from build123d import *

# Parameters (mm, degrees)
ESQUISSE1_R        = 1.6
BOSS_EXTRU_1_DEPTH = 5


with BuildPart() as part:
    # Esquisse1 → Boss.-Extru.1 (new body)
    with BuildSketch(Plane(origin=(0, 0, 0), x_dir=(-1, 0, 0), z_dir=(0, 0, -1))):
        with BuildLine():
            Line((-34.923591431, 50.185646262), (-34.593521354, 46.781705469))
            Line((-34.593521354, 46.781705469), (-33.97698121, 43.895774796))
            Line((-33.97698121, 43.895774796), (-33.105501007, 41.345514202))
            Line((-33.105501007, 41.345514202), (-31.977290744, 38.953213644))
            Line((-31.977290744, 38.953213644), (-31.383990606, 37.884363395))
            Line((-31.383990606, 37.884363395), (-30.617930427, 37.00766319))
            Line((-30.617930427, 37.00766319), (-29.575780184, 36.488623069))
            Line((-29.575780184, 36.488623069), (-28.414519914, 36.40541305))
            Line((-28.414519914, 36.40541305), (-27.309019656, 36.770573135))
            ThreePointArc((-27.309019656, 36.770573135), (-17.618450893, 31.41303394), (-26.770699625, 25.180322464))
            Line((-26.770699625, 25.180322464), (-28.005176529, 25.48125594))
            Line((-28.005176529, 25.48125594), (-29.206336809, 25.243975885))
            Line((-29.206336809, 25.243975885), (-30.212657043, 24.546555722))
            Line((-30.212657043, 24.546555722), (-30.856527193, 23.50514548))
            Line((-30.856527193, 23.50514548), (-32.12730749, 19.451734535))
            Line((-32.12730749, 19.451734535), (-33.010967696, 15.362733581))
            Line((-33.010967696, 15.362733581), (-33.301107763, 13.363943115))
            Line((-33.301107763, 13.363943115), (-33.187947737, 12.109172823))
            Line((-33.187947737, 12.109172823), (-32.569567593, 11.011512567))
            Line((-32.569567593, 11.011512567), (-31.555037356, 10.264542393))
            Line((-31.555037356, 10.264542393), (-30.323257069, 10.000002331))
            Line((-30.323257069, 10.000002331), (-21.600005036, 10.000002331))
            ThreePointArc((-21.600005036, 10.000002331), (-21.246451562, 10.146448975), (-21.100004919, 10.500002448))
            Line((-21.100004919, 10.500002448), (-21.100004919, 14.000002331))
            Line((-21.100004919, 14.000002331), (-22.250004919, 14.000002331))
            ThreePointArc((-22.250004919, 14.000002331), (-22.676781614, 13.823225636), (-22.500004919, 14.250002331))
            Line((-22.500004919, 14.250002331), (-22.500004919, 16.250002331))
            ThreePointArc((-22.500004919, 16.250002331), (-22.676781614, 16.676779027), (-22.250004919, 16.500002331))
            Line((-22.250004919, 16.500002331), (-21.100004919, 16.500002331))
            Line((-21.100004919, 16.500002331), (-21.100004919, 17.750004196))
            ThreePointArc((-21.100004919, 17.750004196), (-21.276780955, 18.176781551), (-20.850004919, 18.000002331))
            Line((-20.850004919, 18.000002331), (-18.450004919, 18.000002331))
            ThreePointArc((-18.450004919, 18.000002331), (-18.023228224, 18.176779027), (-18.200004919, 17.750002331))
            Line((-18.200004919, 17.750002331), (-18.200004919, 16.500002331))
            Line((-18.200004919, 16.500002331), (-17.15000394, 16.500002331))
            ThreePointArc((-17.15000394, 16.500002331), (-16.763072854, 16.709167045), (-16.800004919, 16.270873119))
            Line((-16.800004919, 16.270873119), (-16.800004919, 14.250002331))
            ThreePointArc((-16.800004919, 14.250002331), (-16.623228224, 13.823225636), (-17.050004919, 14.000002331))
            Line((-17.050004919, 14.000002331), (-18.200004919, 14.000002331))
            Line((-18.200004919, 14.000002331), (-18.200004919, 10.500002448))
            ThreePointArc((-18.200004919, 10.500002448), (-18.053558275, 10.146448975), (-17.700004802, 10.000002331))
            Line((-17.700004802, 10.000002331), (-13.900003182, 10.000002331))
            ThreePointArc((-13.900003182, 10.000002331), (-13.473226487, 10.176779027), (-13.650003182, 9.750002331))
            Line((-13.650003182, 9.750002331), (-13.650003182, 0.500000117))
            ThreePointArc((-13.650003182, 0.500000117), (-13.503556539, 0.146446644), (-13.150003066, 0))
            Line((-13.150003066, 0), (-7.150001767, 0))
            ThreePointArc((-7.150001767, 0), (-6.796448223, 0.146446673), (-6.65000155, 0.500000217))
            Line((-6.65000155, 0.500000217), (-6.65000155, 9.750002273))
            Line((-6.65000155, 9.750002273), (-6.775001579, 9.783495281))
            Line((-6.775001579, 9.783495281), (-6.866507601, 9.875002302))
            Line((-6.866507601, 9.875002302), (-6.900001609, 10.000002331))
            Line((-6.900001609, 10.000002331), (-6.866507601, 10.12500236))
            Line((-6.866507601, 10.12500236), (-6.775001579, 10.216512382))
            Line((-6.775001579, 10.216512382), (-6.65000155, 10.25000239))
            Line((-6.65000155, 10.25000239), (-6.525001521, 10.216512382))
            Line((-6.525001521, 10.216512382), (-6.4334955, 10.12500236))
            Line((-6.4334955, 10.12500236), (-6.400001492, 10.000002331))
            Line((-6.400001492, 10.000002331), (-0.500000117, 10.000002331))
            ThreePointArc((-0.500000117, 10.000002331), (-0.146446644, 10.146448975), (0, 10.500002448))
            Line((0, 10.500002448), (0, 15.500002215))
            ThreePointArc((0, 15.500002215), (-0.146446644, 15.853555688), (-0.500000117, 16.000002331))
            Line((-0.500000117, 16.000002331), (-2.461443863, 16.000002331))
            ThreePointArc((-2.461443863, 16.000002331), (-2.814997336, 16.146448975), (-2.96144398, 16.500002448))
            Line((-2.96144398, 16.500002448), (-2.96144398, 47.033035527))
            ThreePointArc((-2.96144398, 47.033035527), (-3.113686629, 47.798409924), (-3.547236949, 48.44726269))
            Line((-3.547236949, 48.44726269), (-6.775657869, 51.67567661))
            ThreePointArc((-6.775657869, 51.67567661), (-7.42450983, 52.109224866), (-8.18988253, 52.261466746))
            Line((-8.18988253, 52.261466746), (-32.925020965, 52.261466746))
            ThreePointArc((-32.925020965, 52.261466746), (-34.365794593, 51.648615258), (-34.923591431, 50.185646262))
        make_face()
        with Locations((-8.611451235, 46.611460467)):
            Circle(ESQUISSE1_R, mode=Mode.SUBTRACT)
        with Locations((-8.650001767, 15.611460467)):
            Circle(ESQUISSE1_R, mode=Mode.SUBTRACT)
        Polygon((-31.600007367, 43.300010094), (-31.566507359, 43.425010123), (-31.475007338, 43.516520145), (-31.350007308, 43.550010153), (-31.350007308, 49.550011551), (-31.475007338, 49.583511559), (-31.566507359, 49.67501158), (-31.600007367, 49.80001161), (-31.566507359, 49.925011639), (-31.475007338, 50.01652166), (-31.350007308, 50.050011668), (-31.225007279, 50.01652166), (-31.133507258, 49.925011639), (-31.10000725, 49.80001161), (-28.400006621, 49.80001161), (-28.366516613, 49.925011639), (-28.275006592, 50.01652166), (-28.150006562, 50.050011668), (-28.025006533, 50.01652166), (-27.933496512, 49.925011639), (-27.900006504, 49.80001161), (-27.933496512, 49.67501158), (-28.025006533, 49.583511559), (-28.150006562, 49.550011551), (-28.150006562, 43.550010153), (-28.025006533, 43.516520145), (-27.933496512, 43.425010123), (-27.900006504, 43.300010094), (-27.933496512, 43.175010065), (-28.025006533, 43.083510044), (-28.150006562, 43.050010036), (-28.275006592, 43.083510044), (-28.366516613, 43.175010065), (-28.400006621, 43.300010094), (-31.10000725, 43.300010094), (-31.133507258, 43.175010065), (-31.225007279, 43.083510044), (-31.350007308, 43.050010036), (-31.475007338, 43.083510044), (-31.566507359, 43.175010065), align=None, mode=Mode.SUBTRACT)
    extrude(amount=-BOSS_EXTRU_1_DEPTH)


solid = part.part
For this review, take the finished solid that the model builds, in its own axes (mm). A direction names the side the tool comes from. Round coordinates to 2 decimals unless told otherwise and drop trailing zeros. Loops run counter-clockwise (first coordinate to the right, second up) from the corner with the lowest first, then second, coordinate; pieces in that order, holes last. Notation, with made-up numbers: (-32.75, 28.5) - (24.25, 28.5) arc R15 cw to (24.25, 55.5) - close; hole circle Ø11 at (68, 89.25). An arc over 180 degrees is marked (long way). One line per item, written item: value. Start each with the question number.
Item 1: Take a section at A-A (y = 8). Give the boundary of the cut face in (x, z).
Item 2: For L1, parallel to Y at x = 24, z = 3.8; L2, parallel to X at y = 46.5, z = 2.1; L3, parallel to X at y = 15, z = 2.8, list the stretches that pass through material, from the lowest coordinate up.
Item 3: Take a section at B-B (z = 3.35). State how many separate pieces and enclosed holes the cut face has, plus the area to 3 significant figures.
Item 4: Clearance check with flat-ended pins moving along their axes: pin 1 Ø1 at (y, z) = (28.5, 2.5) entering from +X; pin 2 Ø4 at (x, y) = (21, 28) entering from +Z; pin 3 Ø1.5 at (x, y) = (18, 25.5) entering from -Z; pin 4 Ø0.8 at (x, z) = (30, 2.5) entering from -Y. State where each tip first meets the part, or that it passes through.
Item 5: The part is to be moulded in two halves that separate along X. For faces 1 (the flat face through (6.65, 5, 2)), 2 (the flat face through (18.2, 17, 2)), 3 (the flat face through (30, 49.8, 2)), 4 (the flat face through (31.685, 38.426, 2.465)), say which applies: +X half, -X half, draft (parallel to the pull), parting line (faces both ways), or undercut.
Item 6: Take a section at C-C (y = 33.5). Give the boundary of the cut face in (x, z), plus the area to 3 significant figures.
Item 7: For faces 5 (the flat face through (22, 14, 2)), 6 (the flat face through (2.961, 32, 2)), 7 (the flat face through (3, 10, 2)), 8 (the flat face through (33.547, 42.638, 2.465)), list the 3-axis set-ups (+Z, -Z, +X, -X, +Y, -Y) from which the entire face can be reached by the end or side of a thin tool; tool diameter is ignored.
Answer below:
1. outline: (6.65, 0) - (13.65, 0) - (13.65, 5) - (6.65, 5) - close
2. L1: y = 10 to 24.61, 37.61 to 52.26
2. L2: x = 2.96 to 7.02, 10.21 to 28.15, 31.35 to 34.53
2. L3: x = 0 to 7.17, 10.13 to 16.8, 22.5 to 33.06
3. separate pieces: 1
3. enclosed holes: 3
3. area: 1,100 mm2
4. pin 1: stops at x = 18.4
4. pin 2: passes through
4. pin 3: stops at z = 0
4. pin 4: stops at y = 10
5. face 1: -X half
5. face 2: undercut
5. face 3: undercut
5. face 4: +X half
6. outline: (2.96, 0) - (18.07, 0) - (18.07, 5) - (2.96, 5) - close
6. area: 75.5 mm2
7. face 5: +Z, -Z
7. face 6: +Z, -Z, -X, +Y
7. face 7: +Z, -Z, -X, -Y
7. face 8: +Z, -Z, +X
